Can you work these out from the model? Positions are in its coordinate system, mm. Face numbers are marked on the shaded views. A direction names the side the tool comes from. Give positions to 0.01 mm unless a question says otherwise; leave off trailing zeros. Loops run counter-clockwise (first coordinate to the right, second up) from the corner with the lowest first, then second, coordinate; pieces in that order, holes last. Notation, with made-up numbers: (36, -34.5) -> (87, -34.5) arc R33 ccw to (87, -5.5) -> close; hole circle Ø6 at (-10, 0). An arc over 180 degrees is marked (long way). Use CSV: the item, a comma, the result in double quotes.
from build123d import *

# Parameters (mm, degrees)
F1_DEPTH  = 76.2
F2_W      = 16.5251810104
F2_H      = 54.9541674554
F1_FACE_W = 76.2
F1_FACE_H = 67.6971774679
F3_DEPTH  = 25.4


with BuildPart() as f1:
    # F0 (on Front) → F1 (new body)
    with BuildSketch(Plane.XZ):
        Polygon((76.2232616544, 0), (37.109632045, 55.2542470396), (0, 0), align=None)
    extrude(amount=F1_DEPTH)

    # F2 (on Right) + F1_face (on face) → F3 (join)
    with BuildSketch(Plane.YZ):
        with Locations((-36.0880820081, 27.4770837277)):
            Rectangle(F2_W, F2_H)
    with BuildSketch(Plane(origin=(56.6664468497, -38.1, 27.6271235198), x_dir=(0, 1, 0), z_dir=(0.8161972051, 0, 0.5777734179))):
        Rectangle(F1_FACE_W, F1_FACE_H)
    extrude(amount=F3_DEPTH, dir=(1, 0, 0))


solid = f1.part
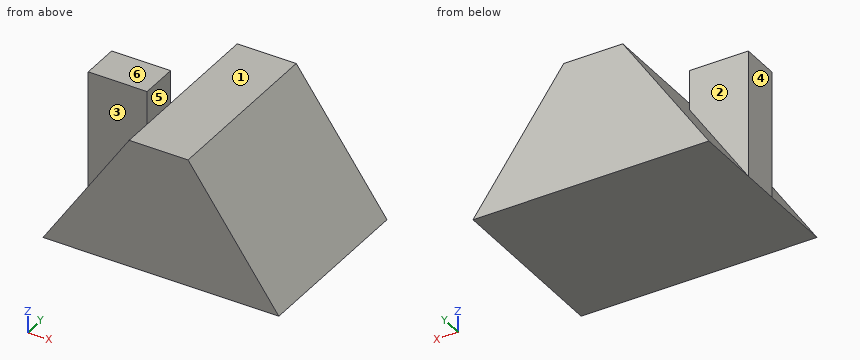
(1) If we section it at A-A, the plane y = -41.5: Write out the boundary of the cut face in (x, z).
Answer sheet:
outline,"(0, 0) -> (101.62, 0) -> (62.51, 55.25) -> (37.11, 55.25) -> (25.4, 37.82) -> (25.4, 54.95) -> (0, 54.95) -> close"
(2) Which directions (+Z, -Z, +X, -X, +Y, -Y) give clear straight access to the entire face, cutting with the end or side of a thin tool? Please do the marked faces 1, 2 and 3.
Answer sheet:
face 1,"+Z, +X, -X, +Y, -Y"
face 2,"+Z, -X, +Y"
face 3,"+Z, -X, -Y"
(3) If we section it at C-C, the plane x = 6: Write out the boundary of the cut face in (y, z), then the cut area to 3 significant figures.
Answer sheet:
outline,"(-76.2, 0) -> (0, 0) -> (0, 8.93) -> (-27.83, 8.93) -> (-27.83, 54.95) -> (-44.35, 54.95) -> (-44.35, 8.93) -> (-76.2, 8.93) -> close"
area,"1,440 mm2"
(4) If I drill on L1, parallel to Y at x = 7, z = 35; L2, parallel to X at y = -25.5, z = 27; L3, parallel to Z at x = 34, y = -62, over which ranges is the centre line in solid material (lowest first)? Write a range as from..to.
Answer sheet:
L1,"y = -44.35..-27.83"
L2,"x = 18.13..82.51"
L3,"z = 0..50.62"
(5) If we section it at B-B, the plane z = 47: Write out the boundary of the cut face in (x, y).
Answer sheet:
outline,"(0, -44.35) -> (25.4, -44.35) -> (25.4, -27.83) -> (0, -27.83) -> close; (31.57, -76.2) -> (68.35, -76.2) -> (68.35, 0) -> (31.57, 0) -> close"
(6) We'd pull the mould along X, two halves only. Please class the marked faces 4, 5 and 6: released by +X, released by -X, zero draft, split by the parting line, or undercut.
Answer sheet:
face 4,"released by -X"
face 5,"undercut"
face 6,"zero draft"
(7) If we section it at D-D, the plane z = 36.5: Write out the boundary of the cut face in (x, y).
Answer sheet:
outline,"(0, -44.35) -> (24.51, -44.35) -> (24.51, -76.2) -> (75.79, -76.2) -> (75.79, 0) -> (24.51, 0) -> (24.51, -27.83) -> (0, -27.83) -> close"
(8) Will these pins go through, and if not, where does the flat tip stop? pin 1 Ø20.5 at (x, z) = (11, 16.5) entering from -Y; pin 2 Ø5 at (x, y) = (14.5, -39) entering from +Z; pin 3 Ø1 at (y, z) = (-16, 34) entering from -X; pin 4 Ø18 at (y, z) = (-40, 50) entering from +X.
Answer sheet:
pin 1,"stops at y = -76.2"
pin 2,"stops at z = 54.95"
pin 3,"stops at x = 22.5"
pin 4,"stops at x = 72.6"
